Source: CAD feature listing. Evaluate the final solid. Frame: model axes, mm. Face numbers are marked on the shaded views. A direction names the side the tool comes from. Give positions to 0.01 mm unless a question says otherwise; leave off trailing zeros. Loops run counter-clockwise (first coordinate to the right, second up) from the corner with the lowest first, then second, coordinate; pieces in that order, holes last.
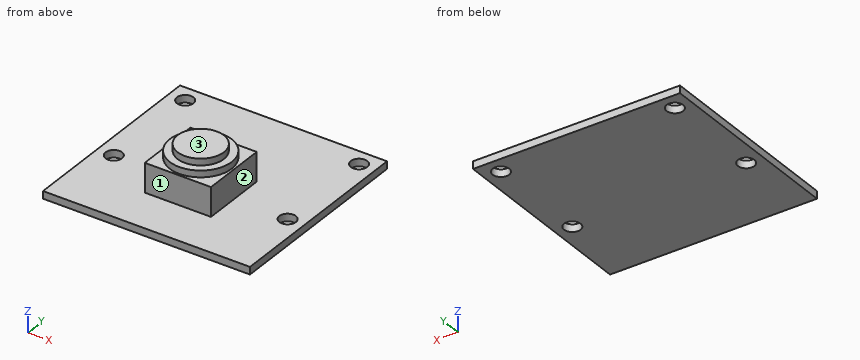
```python
from build123d import *

# Parameters (mm, degrees)
CROQUIS1_W              = 25
CROQUIS1_H              = 24
CROQUIS1_R              = 1
SALIENTE_EXTRUIR1_DEPTH = 0.9
CROQUIS2_W              = 8
CROQUIS2_H              = 8
SALIENTE_EXTRUIR2_DEPTH = 3.5
CROQUIS3_R              = 3.75
SALIENTE_EXTRUIR3_DEPTH = 0.8
CROQUIS4_R              = 2.8
SALIENTE_EXTRUIR4_DEPTH = 0.8


with BuildPart() as part:
    # Croquis1 → Saliente-Extruir1 (new body)
    with BuildSketch(Plane.XY):
        Rectangle(CROQUIS1_W, CROQUIS1_H)
        with Locations((10.5, 10)):
            Circle(CROQUIS1_R, mode=Mode.SUBTRACT)
        with Locations((10.5, -2.5)):
            Circle(CROQUIS1_R, mode=Mode.SUBTRACT)
        with Locations((-10.5, -2.5)):
            Circle(CROQUIS1_R, mode=Mode.SUBTRACT)
        with Locations((-10.5, 10)):
            Circle(CROQUIS1_R, mode=Mode.SUBTRACT)
    extrude(amount=SALIENTE_EXTRUIR1_DEPTH)

    # Croquis2 → Saliente-Extruir2 (add)
    with BuildSketch(Plane.XY.offset(0.9)):
        with Locations((0, -2.5)):
            Rectangle(CROQUIS2_W, CROQUIS2_H)
    extrude(amount=SALIENTE_EXTRUIR2_DEPTH)

    # Croquis3 → Saliente-Extruir3 (add)
    with BuildSketch(Plane.XY.offset(4.4)):
        with Locations((0, -2.5)):
            Circle(CROQUIS3_R)
    extrude(amount=SALIENTE_EXTRUIR3_DEPTH)

    # Croquis4 → Saliente-Extruir4 (add)
    with BuildSketch(Plane.XY.offset(5.2)):
        with Locations((0, -2.5)):
            Circle(CROQUIS4_R)
    extrude(amount=SALIENTE_EXTRUIR4_DEPTH)


solid = part.part
```
(1) Section A-A, the plane x = -10.5. Return the cut outline in (y, z).
A:
outline: (-12, 0) - (-3.5, 0) - (-3.5, 0.9) - (-12, 0.9) - close; (-1.5, 0) - (9, 0) - (9, 0.9) - (-1.5, 0.9) - close; (11, 0) - (12, 0) - (12, 0.9) - (11, 0.9) - close
(2) Section C-C, the plane y = -2.5. Return the cut outline in (x, z), then the cut area to 3 significant figures.
A:
outline: (-12.5, 0) - (-11.5, 0) - (-11.5, 0.9) - (-12.5, 0.9) - close; (-9.5, 0) - (9.5, 0) - (9.5, 0.9) - (4, 0.9) - (4, 4.4) - (3.75, 4.4) - (3.75, 5.2) - (2.8, 5.2) - (2.8, 6) - (-2.8, 6) - (-2.8, 5.2) - (-3.75, 5.2) - (-3.75, 4.4) - (-4, 4.4) - (-4, 0.9) - (-9.5, 0.9) - close; (11.5, 0) - (12.5, 0) - (12.5, 0.9) - (11.5, 0.9) - close
area: 57.4 mm2
(3) Section D-D, the plane x = -0.25. Return the cut outline in (y, z), then the cut area to 3 significant figures.
A:
outline: (-12, 0) - (12, 0) - (12, 0.9) - (1.5, 0.9) - (1.5, 4.4) - (1.24, 4.4) - (1.24, 5.2) - (0.29, 5.2) - (0.29, 6) - (-5.29, 6) - (-5.29, 5.2) - (-6.24, 5.2) - (-6.24, 4.4) - (-6.5, 4.4) - (-6.5, 0.9) - (-12, 0.9) - close
area: 60.0 mm2
(4) First-contact query: pin 1 (1.5 mm diameter, centred on x = 2.5, y = -1, fed in from +Z); pin 2 (1 mm diameter, centred on x = -2, z = 3, fed in from +Y); pin 3 (1 mm diameter, centred on y = -3.5, z = 3, fed in from +X); pin 4 (1 mm diameter, centred on x = 3.5, z = 5, fed in from +Y). Flat tips, straight axial feed; report the tip coordinate or a pass-through.
A:
pin 1: stops at z = 6
pin 2: stops at y = 1.5
pin 3: stops at x = 4
pin 4: stops at y = -0.25
(5) Section B-B, the plane y = 10. Return the cut outline in (x, z).
A:
outline: (-12.5, 0) - (-11.5, 0) - (-11.5, 0.9) - (-12.5, 0.9) - close; (-9.5, 0) - (9.5, 0) - (9.5, 0.9) - (-9.5, 0.9) - close; (11.5, 0) - (12.5, 0) - (12.5, 0.9) - (11.5, 0.9) - close
(6) Ray query, line 1 along Y through (x, z) = (-10.5, 0.75); line 2 along Z through (x, y) = (9, 2); line 3 along Y through (x, z) = (-3, 2.25). Return the intervals inside material, ascending.
A:
line 1: y = -12 to -3.5, -1.5 to 9, 11 to 12
line 2: z = 0 to 0.9
line 3: y = -6.5 to 1.5
(7) Reachability of the marked faces 1, 2 and 3 from +Z, -Z, +X, -X, +Y, -Y: full face, straight path, thin tool, end or side. Return the list, or none.
A:
face 1: +Z, +X, -X, -Y
face 2: +Z, +X, +Y, -Y
face 3: +Z, +X, -X, +Y, -Y
